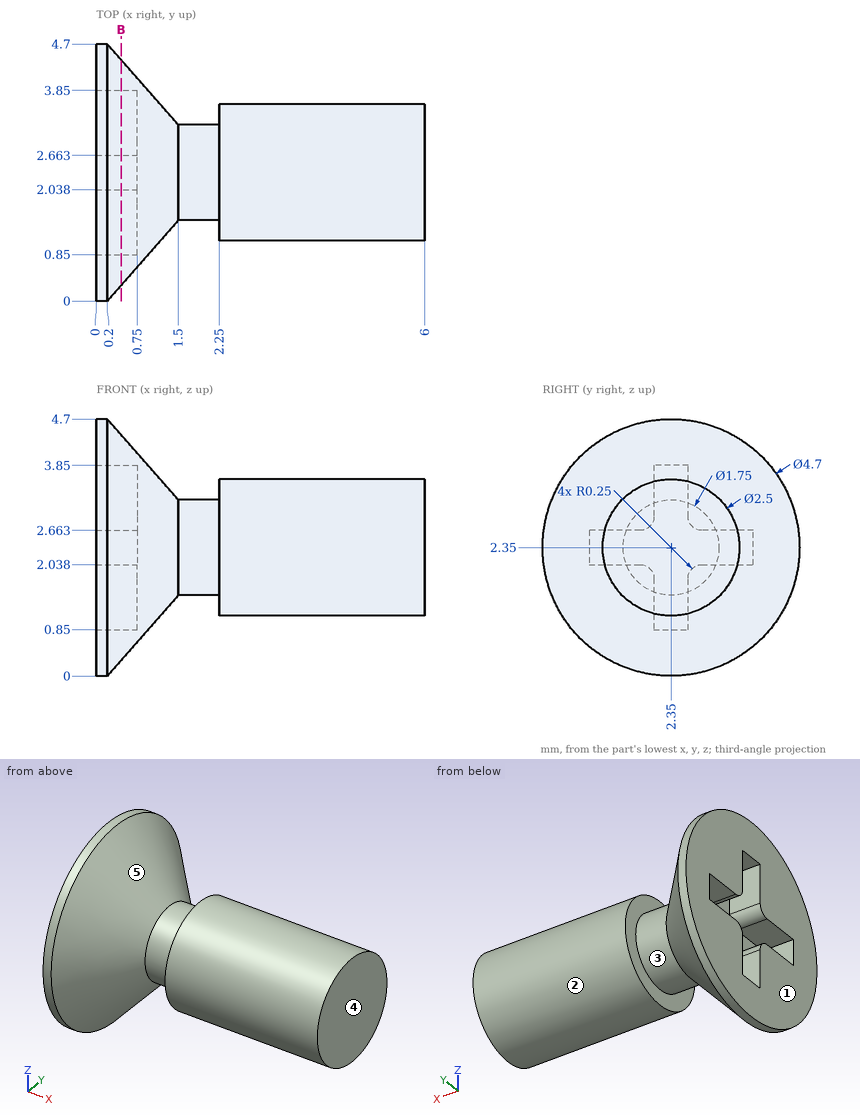
Part print with two shaded views. Sizes in mm from the minimum x, y, z corner. A direction names the side the tool comes from. Round coordinates to 2 decimals unless told otherwise and drop trailing zeros. Write each loop counter-clockwise with the first axis right and the second up, starting at its lowest first coordinate (ties: lowest second). Pieces come first, ordered by that corner, then holes. Notation, with made-up numbers: (89.5, 76) -> (136.5, 76) arc R17 cw to (136.5, 90) -> close; hole circle Ø7 at (61, 34.5). An arc over 180 degrees is marked (long way). Use one line per item in the form item = value.
Q1. Band-saw the part on B-B, the plane x = 0.45. Write the cut outline in (y, z).
Conclusion:
outline = circle Ø4.13 at (2.35, 2.35); hole (0.85, 2.04) -> (1.79, 2.04) arc R0.25 cw to (2.04, 1.79) -> (2.04, 0.85) -> (2.66, 0.85) -> (2.66, 1.79) arc R0.25 cw to (2.91, 2.04) -> (3.85, 2.04) -> (3.85, 2.66) -> (2.91, 2.66) arc R0.25 cw to (2.66, 2.91) -> (2.66, 3.85) -> (2.04, 3.85) -> (2.04, 2.91) arc R0.25 cw to (1.79, 2.66) -> (0.85, 2.66) -> close
Q2. Drill centre lines: L1, parallel to X at y = 2.4, z = 1.95; L2, parallel to Y at x = 5.65, z = 2.3; L3, parallel to X at y = 2.55, z = 0.3 (1 decimal). Where is each one in solid material? Low to high.
Conclusion:
L1 = 0.75 to 6
L2 = 1.1 to 3.6
L3 = 0 to 0.5
Q3. Two-plate mould, pull along X, no slides. Class the marked faces 1, 2 and 3: released by +X, released by -X, zero draft, split by the parting line, or undercut.
Conclusion:
face_1 = released by -X
face_2 = zero draft
face_3 = undercut
Q4. Drop flat-ended pins along their axis: P1, Ø0.8, axis at x = 0.5, z = 1.5, coming from the +Y side (1 decimal); P2, Ø2, axis at x = 5, z = 1, coming from the -Y side; P3, Ø0.6, axis at x = 0.5, z = 1.5, coming from the -Y side (1 decimal). Give the stop position or say it passes through.
Conclusion:
P1 = 4.6
P2 = 1.15
P3 = 0.1
Q5. Tool access for the marked faces 4 and 5: list every direction of +Z, -Z, +X, -X, +Y, -Y with a clear straight run to the whole face (end or side of a thin tool).
Conclusion:
face_4 = +Z, -Z, +X, +Y, -Y
face_5 = none
